from build123d import *

# Parameters (mm, degrees)
SKETCH1_R           = 9.525
BOSS_EXTRUDE1_DEPTH = 3.175
SKETCH2_R           = 6.35
BOSS_EXTRUDE2_DEPTH = 4.064
SKETCH3_R           = 5.715
BOSS_EXTRUDE3_DEPTH = 15.875
SKETCH4_R           = 4.1275
CUT_EXTRUDE1_DEPTH  = 27.752724086
SKETCH5_W           = 12.7
SKETCH5_H           = 2.54
CUT_EXTRUDE2_DEPTH  = 9.525
CUT_EXTRUDE4_START  = -0.762
SKETCH7_R           = 9.525
SKETCH7_R_2         = 7.112
CUT_EXTRUDE4_DEPTH  = 0.762


with BuildPart() as part:
    # Sketch1 → Boss-Extrude1 (new body)
    with BuildSketch(Plane.XY):
        Circle(SKETCH1_R)
    extrude(amount=BOSS_EXTRUDE1_DEPTH)

    # Sketch2 → Boss-Extrude2 (add)
    with BuildSketch(Plane.XY.offset(3.175)):
        Circle(SKETCH2_R)
    extrude(amount=BOSS_EXTRUDE2_DEPTH)

    # Sketch3 → Boss-Extrude3 (add)
    with BuildSketch(Plane.XY.offset(7.239)):
        Circle(SKETCH3_R)
    extrude(amount=BOSS_EXTRUDE3_DEPTH)

    # Sketch4 → Cut-Extrude1 (cut, through all)
    with BuildSketch(Plane.XY.offset(23.114)):
        Circle(SKETCH4_R)
    extrude(amount=-CUT_EXTRUDE1_DEPTH, mode=Mode.SUBTRACT)

    # Sketch5 → Cut-Extrude2 (cut, symmetric)
    with BuildSketch(Plane(origin=(0, 0, 0), x_dir=(0, 0, -1), z_dir=(1, 0, 0))):
        with Locations((-16.764, 0)):
            Rectangle(SKETCH5_W, SKETCH5_H)
        with BuildLine():
            ThreePointArc((-10.414, 1.27), (-9.144, 0), (-10.414, -1.27))
            Line((-10.414, -1.27), (-10.414, 1.27))
        make_face()
    extrude(amount=CUT_EXTRUDE2_DEPTH, both=True, mode=Mode.SUBTRACT)

    # Sketch7 → Cut-Extrude4 (cut)
    with BuildSketch(Plane.XY.offset(3.175).offset(CUT_EXTRUDE4_START)):
        Circle(SKETCH7_R)
        Circle(SKETCH7_R_2, mode=Mode.SUBTRACT)
    extrude(amount=CUT_EXTRUDE4_DEPTH, mode=Mode.SUBTRACT)


solid = part.part
Design review of the part built by this model. Coordinates are the model's own, in mm. A direction names the side the tool comes from. Give positions to 0.01 mm unless a question says otherwise; leave off trailing zeros. Loops run counter-clockwise (first coordinate to the right, second up) from the corner with the lowest first, then second, coordinate; pieces in that order, holes last. Notation, with made-up numbers: M -19,-8.75 L 1,-8.75 A32 cw 1,19.25 Z; hole C 45.25,23.25 d1. An arc over 180 degrees is marked long. Answer as a JSON object with one key per item and string values.
Item 1: Machinability: for faces 4 (the face through (5, -1.27, 17)), 5 (the face through (-1.38, -6.2, 5.18)), 6 (the face through (0, 5, 23.114)), which of the approach directions +Z, -Z, +X, -X, +Y, -Y give a long, thin tool a straight path to every point of the face, cutting with its end or side? Answer none if there is none.
Output values:
{"face 4": "+Z, +X, -X", "face 5": "+Z", "face 6": "+Z, +X, -X, +Y, -Y"}
Item 2: We need section C-C (z = 21). State the section outline as (x, y) points (1 decimal), and give its area (3 significant figures).
Output values:
{"outline": "M -5.6,-1.3 A5.7 ccw 5.6,-1.3 L 3.9,-1.3 A4.1 cw -3.9,-1.3 Z; M -5.6,1.3 L -3.9,1.3 A4.1 cw 3.9,1.3 L 5.6,1.3 A5.7 ccw Z", "area": "40.9 mm2"}
Item 3: Mouldability with a two-part tool opening along Y and no side actions: class faces 1 (the face through (-4.809, 0.028, 9.144)), 2 (the face through (-0.1, -4.4, 23.114)), 3 (the face through (5.45, 1.72, 15.07)) as pulls with the +Y half, pulls with the -Y half, needs draft (parallel to the pull), parting line crosses it, or undercut.
Output values:
{"face 1": "undercut", "face 2": "needs draft", "face 3": "parting line crosses it"}
Item 4: We need section D-D (x = 6). State the section outline as (y, z) points (3 decimals).
Output values:
{"outline": "M -7.398,0 L 7.398,0 L 7.398,2.413 L 3.818,2.413 L 3.818,3.175 L 2.079,3.175 L 2.079,7.239 L -2.079,7.239 L -2.079,3.175 L -3.818,3.175 L -3.818,2.413 L -7.398,2.413 Z"}
Item 5: For P1, Ø3, axis at x = -1, z = 14.5, coming from the +Y side (3 decimals); P2, Ø3, axis at x = -5.5, y = 2.5, coming from the -Z side; P3, Ø1.3, axis at x = -5, z = 19, coming from the +Y side; P4, Ø2, axis at x = 0.5, z = 11, coming from the -Y side (3 decimals), all flat-tipped, find the tip position at first contact; note any pin that passes through.
Output values:
{"P1": "stops at y = 5.715", "P2": "stops at z = 0", "P3": "stops at y = 3.71", "P4": "stops at y = -5.715"}
Item 6: Wall thickness on line 1 along Y through (x, z) = (0, 6.5); line 2 along Y through (x, z) = (0, 14) (1 decimal); line 3 along Z through (x, y) = (-4.25, 4.5): over which ranges is each line inside the solid? List them lowest first.
Output values:
{"line 1": "y = -6.35 to -4.13, 4.13 to 6.35", "line 2": "y = -5.7 to -4.1, 4.1 to 5.7", "line 3": "z = 0 to 7.24"}
